Part model, mm, in its own coordinate system. Round coordinates to 2 decimals unless told otherwise and drop trailing zeros. Order: outer loops, then holes, each group sorted by start corner. A loop starts at its lowest first (then second) coordinate and runs counter-clockwise, first axis right, second up. Notation, with made-up numbers: (56, -6.5) -> (64, -6.5) arc R34 cw to (64, 30.5) -> close; hole circle Ø5 at (24, -0.5). An arc over 180 degrees is marked (long way). Answer as a JSON object with one key per item and string values. Group by question number.
```python
from build123d import *

# Parameters (mm, degrees)
F0_W      = 80.8181799948
F0_H      = 39.9472732097
F1_DEPTH  = 5.588
F2_W      = 6.1383359134
F2_H      = 6.141224876
F3_DEPTH  = 22.098
F2_H_2    = 7.1644689888
F4_DEPTH  = 22.86
F2_W_2    = 6.2832608819
F5_DEPTH  = 21.59
F6_DEPTH  = 23.114
F7_W      = 3.141630441
F7_H      = 3.070612438
F8_DEPTH  = 18.542
F9_DEPTH  = 25.4
F11_W     = 3.5289935768
F11_H     = 3.6606490612
F13_DEPTH = 19.304
F14_DEPTH = 27.432
F15_DEPTH = 44.958
F12_W     = 3.1885020435
F12_H     = 3.5822344944
F16_DEPTH = 19.812


with BuildPart() as f1:
    # F0 (on Top) → F1 (new body)
    with BuildSketch(Plane.XY):
        with Locations((-2.7709100395, -2.3090904579)):
            Rectangle(F0_W, F0_H)
    extrude(amount=F1_DEPTH)

    # F2 (on face) → F3 (join)
    with BuildSketch(Plane(origin=(0, 0, 0), x_dir=(1, 0, 0), z_dir=(0, 0, -1))):
        with Locations((-40.1108320802, 19.2121146247)):
            Rectangle(F2_W, F2_H)
    extrude(amount=F3_DEPTH)

    # F2 (on face) → F4 (join)
    with BuildSketch(Plane(origin=(0, 0, 0), x_dir=(1, 0, 0), z_dir=(0, 0, -1))):
        with Locations((-40.1108320802, -14.0823116526)):
            Rectangle(F2_W, F2_H_2)
    extrude(amount=F4_DEPTH)

    # F2 (on face) → F5 (join)
    with BuildSketch(Plane(origin=(0, 0, 0), x_dir=(1, 0, 0), z_dir=(0, 0, -1))):
        with Locations((34.4965495169, 19.2121146247)):
            Rectangle(F2_W_2, F2_H)
    extrude(amount=F5_DEPTH)

    # F2 (on face) → F6 (join)
    with BuildSketch(Plane(origin=(0, 0, 0), x_dir=(1, 0, 0), z_dir=(0, 0, -1))):
        with Locations((34.4965495169, -14.0823116526)):
            Rectangle(F2_W_2, F2_H_2)
    extrude(amount=F6_DEPTH)

    # F7 (on face) → F8 (cut)
    with BuildSketch(Plane(origin=(0, 0, -21.59), x_dir=(1, 0, 0), z_dir=(0, 0, -1))):
        with Locations((32.9257342964, 17.6768084057)):
            Rectangle(F7_W, F7_H)
    extrude(amount=-F8_DEPTH, mode=Mode.SUBTRACT)

    # F9 (add): a face of the model
    f9_faces = [f1.faces().sort_by_distance(p)[0] for p in [
        (34.4965495169, 14.0823116526, -23.114),
    ]]
    extrude(f9_faces, amount=F9_DEPTH)

    # F11 (on face) → F13 (cut)
    with BuildSketch(Plane(origin=(0, 0, -22.098), x_dir=(1, 0, 0), z_dir=(0, 0, -1))):
        with Locations((-38.8061609119, 17.9718267173)):
            Rectangle(F11_W, F11_H)
    extrude(amount=-F13_DEPTH, mode=Mode.SUBTRACT)

    # F10 (on face) → F14 (cut)
    with BuildSketch(Plane(origin=(0, 0, -48.514), x_dir=(1, 0, 0), z_dir=(0, 0, -1))):
        Polygon((37.6381799579, -10.5000771582), (34.951556474, -10.5000771582), (34.951556474, -14.6074714139), (31.354919076, -14.6074714139), (31.354919076, -17.664546147), (37.6381799579, -17.664546147), align=None)
    extrude(amount=-F14_DEPTH, mode=Mode.SUBTRACT)

    # F15 (cut): a face of the model
    f15_faces = [f1.faces().sort_by_distance(p)[0] for p in [
        (33.153237775, 12.5537742861, -48.514),
    ]]
    extrude(f15_faces, amount=-F15_DEPTH, mode=Mode.SUBTRACT)

    # F12 (on face) → F16 (cut)
    with BuildSketch(Plane(origin=(0, 0, -22.86), x_dir=(1, 0, 0), z_dir=(0, 0, -1))):
        with Locations((-38.6359151453, -12.2911944054)):
            Rectangle(F12_W, F12_H)
    extrude(amount=-F16_DEPTH, mode=Mode.SUBTRACT)


solid = f1.part
```
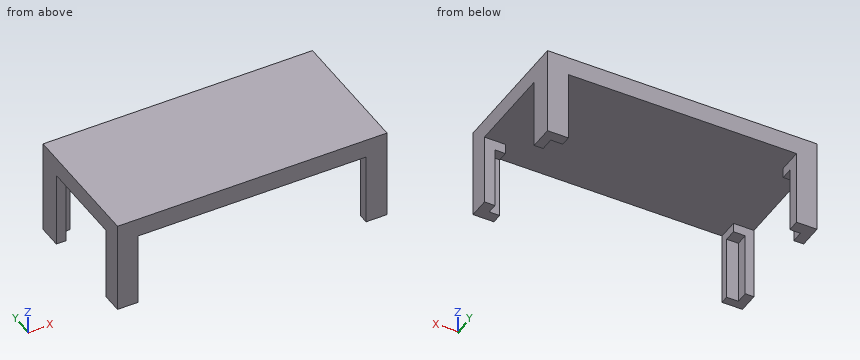
Q1. Band-saw the part on B-B (y = 12.5). List the corners of the cut face in (x, z).
Q2. Wall check: line 1 (X direction, y = -19.5, z = -5.75); line 2 (X direction, y = -20, z = -3); line 3 (Y direction, x = 33, z = -2.5). Give the ranges that are in metal, low to high. Write a range as [from, to].
Q3. Band-saw the part on A-A (z = -19.75). List the corners of the cut face in (x, y).
Q4. Band-saw the part on D-D (y = -18). List the corners of the cut face in (x, z), plus the area to 3 significant figures.
Q5. Band-saw the part on C-C (x = 23.5). List the corners of the cut face in (y, z).
Q6. Drop flat-ended pins along their axis: pin 1 Ø5 at (x, y) = (34, 15) entering from -Z; pin 2 Ø4 at (x, y) = (-39, -18.5) entering from -Z; pin 3 Ø1 at (x, y) = (-2, -10) entering from -Z. Give the stop position or say it passes through.
Completed:
{
 "1": {"outline": "(-43.18, -22.86) -> (-40.23, -22.86) -> (-40.23, -3.05) -> (-37.04, -3.05) -> (-37.04, 0) -> (31.35, 0) -> (31.35, -3.56) -> (34.95, -3.56) -> (34.95, -21.08) -> (37.64, -21.08) -> (37.64, 5.59) -> (-43.18, 5.59) -> close"},
 "2": {"line 1": "[-43.18, -40.57], [31.35, 37.64]", "line 2": "[-43.18, -37.04], [31.35, 37.64]", "line 3": "[-22.28, -16.14], [10.5, 17.66]"},
 "3": {"outline": "(-43.18, -22.28) -> (-37.04, -22.28) -> (-37.04, -19.8) -> (-40.57, -19.8) -> (-40.57, -16.14) -> (-43.18, -16.14) -> close; (-43.18, 10.5) -> (-40.23, 10.5) -> (-40.23, 14.08) -> (-37.04, 14.08) -> (-37.04, 17.66) -> (-43.18, 17.66) -> close; (31.35, -22.28) -> (37.64, -22.28) -> (37.64, -16.14) -> (34.5, -16.14) -> (34.5, -19.21) -> (31.35, -19.21) -> close; (31.35, 14.61) -> (34.95, 14.61) -> (34.95, 10.5) -> (37.64, 10.5) -> (37.64, 17.66) -> (31.35, 17.66) -> close"},
 "4": {"outline": "(-43.18, -22.1) -> (-40.57, -22.1) -> (-40.57, -2.79) -> (-37.04, -2.79) -> (-37.04, 0) -> (31.35, 0) -> (31.35, -3.05) -> (34.5, -3.05) -> (34.5, -21.59) -> (37.64, -21.59) -> (37.64, 5.59) -> (-43.18, 5.59) -> close", "area": "597 mm2"},
 "5": {"outline": "(-22.28, 0) -> (17.66, 0) -> (17.66, 5.59) -> (-22.28, 5.59) -> close"},
 "6": {"pin 1": "z = -21.08", "pin 2": "z = -22.1", "pin 3": "z = 0"}
}
